from build123d import *

# Parameters (mm, degrees)
SKETCH1_R                         = 31.75
HEX_AXEL_CUTOUT_OUTSIDE_RIM_DEPTH = 15.875
SKETCH3_R                         = 31.75
SKETCH3_R_2                       = 28.067
PIPE_STEP_DEPTH                   = 2.54
SKETCH5_R                         = 24.892
SKETCH5_R_2                       = 9.525
SPOKE_STEP_DEPTH                  = 2.54
SLOTS_DEPTH                       = 14.335
FILLET1_R                         = 1.27
SKETCH7_W                         = 163.08703459
SKETCH7_H                         = 168.65885573
MIDCUT_DEPTH                      = 8.9375


with BuildPart() as part:
    # Sketch1 → Hex Axel Cutout & Outside Rim (new body)
    with BuildSketch(Plane.XY):
        Circle(SKETCH1_R)
        Polygon((-7.478995387, 0), (-3.739497694, -6.477), (3.739497694, -6.477), (7.478995387, 0), (3.739497694, 6.477), (-3.739497694, 6.477), align=None, mode=Mode.SUBTRACT)
    extrude(amount=HEX_AXEL_CUTOUT_OUTSIDE_RIM_DEPTH)

    # Sketch3 → Pipe Step (cut)
    with BuildSketch(Plane.XY.offset(15.875)):
        Circle(SKETCH3_R)
        Circle(SKETCH3_R_2, mode=Mode.SUBTRACT)
    pipe_step = extrude(amount=-PIPE_STEP_DEPTH, mode=Mode.SUBTRACT)

    # Step Mirror: Pipe Step across plane
    add(pipe_step.mirror(Plane.XY.offset(7.9375)), mode=Mode.SUBTRACT)

    # Sketch4 → Poly Cord Groove (revolve, cut)
    with BuildSketch(Plane(origin=(0, 0, 0), x_dir=(0, 0, -1), z_dir=(1, 0, 0))):
        with BuildLine():
            Line((-4.7625, 31.75), (-11.1125, 31.75))
            ThreePointArc((-11.1125, 31.75), (-7.9375, 29.21), (-4.7625, 31.75))
        make_face()
    revolve(axis=Axis((0, 0, 13.335), (0, 0, -1)), mode=Mode.SUBTRACT)

    # Sketch5 → Spoke Step (cut)
    with BuildSketch(Plane(origin=(0, 0, 0), x_dir=(-1, 0, 0), z_dir=(0, 0, -1))):
        Circle(SKETCH5_R)
        Circle(SKETCH5_R_2, mode=Mode.SUBTRACT)
    spoke_step = extrude(amount=-SPOKE_STEP_DEPTH, mode=Mode.SUBTRACT)

    # Spoke Step Mirror: Spoke Step across plane
    add(spoke_step.mirror(Plane.XY.offset(7.9375)), mode=Mode.SUBTRACT)

    # Sketch6 → Slots (cut, through all)
    with BuildSketch(Plane.XY.offset(13.335)):
        with BuildLine():
            ThreePointArc((19.589209778, -8.218410987), (21.243338223, 0), (19.589209778, 8.218410987))
            ThreePointArc((19.589209778, 8.218410987), (14.307589254, 10.378115507), (12.147884733, 5.096494983))
            ThreePointArc((12.147884733, 5.096494983), (13.173661777, 0), (12.147884733, -5.096494983))
            ThreePointArc((12.147884733, -5.096494983), (14.307589254, -10.378115507), (19.589209778, -8.218410987))
        make_face()
        with BuildLine():
            ThreePointArc((-8.218410987, -19.589209778), (0, -21.243338223), (8.218410987, -19.589209778))
            ThreePointArc((8.218410987, -19.589209778), (10.378115507, -14.307589254), (5.096494983, -12.147884733))
            ThreePointArc((5.096494983, -12.147884733), (0, -13.173661777), (-5.096494983, -12.147884733))
            ThreePointArc((-5.096494983, -12.147884733), (-10.378115507, -14.307589254), (-8.218410987, -19.589209778))
        make_face()
        with BuildLine():
            ThreePointArc((-19.589209778, 8.218410987), (-21.243338223, 0), (-19.589209778, -8.218410987))
            ThreePointArc((-19.589209778, -8.218410987), (-14.307589254, -10.378115507), (-12.147884733, -5.096494983))
            ThreePointArc((-12.147884733, -5.096494983), (-13.173661777, 0), (-12.147884733, 5.096494983))
            ThreePointArc((-12.147884733, 5.096494983), (-14.307589254, 10.378115507), (-19.589209778, 8.218410987))
        make_face()
        with BuildLine():
            ThreePointArc((8.218410987, 19.589209778), (0, 21.243338223), (-8.218410987, 19.589209778))
            ThreePointArc((-8.218410987, 19.589209778), (-10.378115507, 14.307589254), (-5.096494983, 12.147884733))
            ThreePointArc((-5.096494983, 12.147884733), (0, 13.173661777), (5.096494983, 12.147884733))
            ThreePointArc((5.096494983, 12.147884733), (10.378115507, 14.307589254), (8.218410987, 19.589209778))
        make_face()
    extrude(amount=-SLOTS_DEPTH, mode=Mode.SUBTRACT)

    # Fillet1
    fillet1_edges = [part.edges().sort_by_distance(p)[0] for p in [
        (24.892, 0, 2.54),
        (9.525, 0, 2.54),
        (24.892, 0, 13.335),
        (9.525, 0, 13.335),
    ]]
    fillet(fillet1_edges, radius=FILLET1_R)

    # Sketch7 → MidCut (cut, through all)
    with BuildSketch(Plane.XY.offset(7.9375)):
        with Locations((2.006221024, 3.627486548)):
            Rectangle(SKETCH7_W, SKETCH7_H)
    extrude(amount=-MIDCUT_DEPTH, mode=Mode.SUBTRACT)


solid = part.part
Geometry: final body of the model. Coordinates: model frame, mm. A direction names the side the tool comes from. Round coordinates to 2 decimals unless told otherwise and drop trailing zeros. Order: outer loops, then holes, each group sorted by start corner. A loop starts at its lowest first (then second) coordinate and runs counter-clockwise, first axis right, second up. Notation, with made-up numbers: (4, 46.25) - (52, 46.25) arc R26 cw to (52, 71.25) - close; hole circle Ø2 at (67, 78). An arc over 180 degrees is marked (long way). Write each question's results on one line, items separated by ' | '.
Item 1: Mould query, pull axis X, two halves, no side actions, for faces 4 (the flat face through (-2, -25, 15.875)), 5 (the cylindrical face through (29.33, -12.16, 12.21)), 6 (the cylindrical face through (-21.243, 0.118, 10.674)). Classes: pulls with the +X half, pulls with the -X half, needs draft (parallel to the pull), parting line crosses it, or undercut.
Completed:
face 4: needs draft | face 5: parting line crosses it | face 6: undercut
Item 2: First-contact query: pin 1 Ø2 at (x, z) = (1.5, 10.5) entering from +Y; pin 2 Ø1 at (y, z) = (18.5, 9.5) entering from +X; pin 3 Ø2 at (x, y) = (23, -3.5) entering from +Z. Flat tips, straight axial feed; report the tip coordinate or a pass-through.
Completed:
pin 1: y = 31.74 | pin 2: x = 23.68 | pin 3: z = 13.51
Item 3: Section B-B, the plane z = 12. Return the cut outline in (x, y), and give its area (3 significant figures).
Completed:
outline: circle Ø63.5 at (0, 0); hole (-19.59, -8.22) arc R4.03 ccw to (-12.15, -5.1) arc R13.17 cw to (-12.15, 5.1) arc R4.03 ccw to (-19.59, 8.22) arc R21.24 ccw to start; hole (-8.22, -19.59) arc R21.24 ccw to (8.22, -19.59) arc R4.03 ccw to (5.1, -12.15) arc R13.17 cw to (-5.1, -12.15) arc R4.03 ccw to start; hole (-8.22, 19.59) arc R4.03 ccw to (-5.1, 12.15) arc R13.17 cw to (5.1, 12.15) arc R4.03 ccw to (8.22, 19.59) arc R21.24 ccw to start; hole (-7.48, 0) - (-3.74, -6.48) - (3.74, -6.48) - (7.48, 0) - (3.74, 6.48) - (-3.74, 6.48) - close; hole (12.15, -5.1) arc R4.03 ccw to (19.59, -8.22) arc R21.24 ccw to (19.59, 8.22) arc R4.03 ccw to (12.15, 5.1) arc R13.17 cw to start | area: 2,380 mm^2
Item 4: Section A-A, the plane x = 0. State how many separate pieces and enclosed holes the cut face has, and give its area (3 significant figures).
Completed:
separate pieces: 4 | enclosed holes: 0 | area: 207 mm^2
Item 5: Material intervals for line 1 along Y through (x, z) = (0, 15.6) (3 decimals); line 2 along Y through (x, z) = (7, 10.75); line 3 along X through (y, z) = (10, 9), sorted ascending. Write a range as [from, to].
Completed:
line 1: [-28.067, -24.892], [-9.525, -6.477], [6.477, 9.525], [24.892, 28.067] | line 2: [-30.02, -20.06], [-11.85, -0.83], [0.83, 11.85], [20.06, 30.02] | line 3: [-27.63, -18.13], [-13.61, 13.61], [18.13, 27.63]
Item 6: Reachability of faces 1 (the cylindrical face through (5.4, -24.3, 15.2)), 2 (the cylindrical face through (21.243, -0.118, 10.674)), 3 (the flat face through (6, -6, 7.938)) from +Z, -Z, +X, -X, +Y, -Y: full face, straight path, thin tool, end or side. Return the list, or none.
Completed:
face 1: +Z | face 2: +Z, -Z | face 3: -Z, +X, -X, +Y, -Y
